Autodesk Inventor part; units mm, degrees
ref_plane "YZ Plane" through (0, 0, 0) normal (1, 0, 0) x (0, 1, 0)
ref_plane "XZ Plane" through (0, 0, 0) normal (0, 1, 0) x (-1, 0, 0)
ref_plane "XY Plane" through (0, 0, 0) normal (0, 0, 1) x (1, 0, 0)
sketch "Sketch1" plane through (0, 0, 0) normal (0, 0, 1) x (1, 0, 0)
  line L0 (-17.5, 17.5) -> (17.5, 17.5)
  line L1 (17.5, 17.5) -> (17.5, -17.5)
  line L2 (17.5, -17.5) -> (-17.5, -17.5)
  line L3 (-17.5, -17.5) -> (-17.5, 17.5)
  line L4 (14.5, 14.5) -> (-14.5, 14.5)
  line L5 (-14.5, 14.5) -> (-14.5, -14.5)
  line L6 (-14.5, -14.5) -> (14.5, -14.5)
  line L7 (14.5, -14.5) -> (14.5, 14.5)
  point P0 (0, 0)
  point P1 (17.5, 0)
  point P2 (0, 17.5)
  dimension "d0" = 35
  dimension "d1" = 35
  dimension "d2" = 3
extrude "Extrusion1" add sketch "Sketch1" against normal mid plane 45
chamfer "Chamfer1" distance 2 angle 45 8 edges at (-17.5, 17.5, 0) (17.5, 17.5, 0) (-14.5, 14.5, 0) (14.5, 14.5, 0) (-14.5, -14.5, 0) (14.5, -14.5, 0) (17.5, -17.5, 0) (-17.5, -17.5, 0)
sketch "Sketch2" plane through (0, 0, 22.5) normal (0, 0, 1) x (1, 0, 0)
  line L0 (15.5, 17.5) -> (-15.5, 17.5)
  line L1 (-12.5, 14.5) -> (12.5, 14.5)
  line L2 (-17.5, 15.5) -> (-15.5, 17.5)
  line L3 (-12.5, 14.5) -> (-14.5, 12.5)
  line L4 (14.5, 12.5) -> (12.5, 14.5)
  line L5 (15.5, 17.5) -> (17.5, 15.5)
  line L6 (-17.5, 15.5) -> (-17.5, -15.5)
  line L7 (-14.5, -12.5) -> (-14.5, 12.5)
  line L8 (-14.5, -12.5) -> (-12.5, -14.5)
  line L9 (-15.5, -17.5) -> (15.5, -17.5)
  line L10 (17.5, -15.5) -> (17.5, 15.5)
  line L11 (-15.5, -17.5) -> (-17.5, -15.5)
  line L12 (12.5, -14.5) -> (-12.5, -14.5)
  point P0 (0, 0)
  point P1 (-15, 15)
  point P2 (15, 15)
  point P3 (15, -15)
  point P4 (-15, -17.5)
  point P5 (-15, -15)
  point P6 (15, -17.5)
  dimension "d8" = 3
  dimension "d9" = 4.2426
  dimension "d10" = 2.1213
  dimension "d11" = 5
  dimension "d12" = 2.5
  dimension "d13" = 2.5
  dimension "d14" = 4.2426
  dimension "d15" = 2.1213
  dimension "d26" = 5
  dimension "d27" = 2.5
  dimension "d28" = 5
  dimension "d29" = 2.5
  dimension "d30" = 2.5
  dimension "d31" = 2.5
  dimension "d64" = 4.2426
hole "Hole1" at (-15, 15, 22.5) at (15, 15, 22.5) at (15, -15, 22.5) at (-15, -15, 22.5) direction (0, 0, -1) diameter 2.459 depth 8.8 tip angle 118
sketch "Sketch4" plane through (0, 0, -22.5) normal (0, 0, -1) x (-1, 0, 0)
  line L0 (15.5, 17.5) -> (-15.5, 17.5)
  line L1 (-12.5, 14.5) -> (12.5, 14.5)
  line L2 (-17.5, 15.5) -> (-15.5, 17.5)
  line L3 (-12.5, 14.5) -> (-14.5, 12.5)
  line L4 (14.5, 12.5) -> (12.5, 14.5)
  line L5 (15.5, 17.5) -> (17.5, 15.5)
  line L6 (-17.5, 15.5) -> (-17.5, -17.5)
  line L7 (-14.5, -12.5) -> (-14.5, 12.5)
  line L8 (-14.5, -12.5) -> (-12.5, -14.5)
  line L9 (-17.5, -17.5) -> (17.5, -17.5)
  line L10 (17.5, -17.5) -> (17.5, 15.5)
  line L11 (-17.5, 15.5) -> (-15.5, 17.5)
  line L12 (-17.5, 15.5) -> (-17.5, -15.5)
  line L13 (-15.5, -17.5) -> (15.5, -17.5)
  line L14 (17.5, -15.5) -> (17.5, 15.5)
  line L15 (15.5, 17.5) -> (17.5, 15.5)
  line L16 (15.5, 17.5) -> (-15.5, 17.5)
  line L17 (-14.5, -12.5) -> (-14.5, 12.5)
  line L18 (-12.5, 14.5) -> (-14.5, 12.5)
  line L19 (-12.5, 14.5) -> (12.5, 14.5)
  line L20 (14.5, 12.5) -> (12.5, 14.5)
  line L21 (14.5, 12.5) -> (14.5, -12.5)
  line L22 (12.5, -14.5) -> (14.5, -12.5)
  line L23 (12.5, -14.5) -> (-12.5, -14.5)
  line L24 (-14.5, -12.5) -> (-12.5, -14.5)
  line L25 (17.5, -15.5) -> (15.5, -17.5)
  line L26 (-15.5, -17.5) -> (-17.5, -15.5)
  point P0 (0, 0)
  point P1 (0, 0)
  point P2 (-15, 15)
  point P3 (15, 15)
  point P4 (15, -15)
  point P5 (-15, -15)
  dimension "d39" = 3
  dimension "d40" = 4.2426
  dimension "d41" = 2.1213
  dimension "d42" = 5
  dimension "d43" = 2.5
  dimension "d44" = 2.5
  dimension "d45" = 4.2426
  dimension "d46" = 2.1213
  dimension "d47" = 5.6569
  dimension "d48" = 5
  dimension "d49" = 2.5
  dimension "d50" = 5
  dimension "d51" = 2.5
  dimension "d52" = 2.5
  dimension "d53" = 2.5
hole "Hole2" at (15, 15, -22.5) at (-15, 15, -22.5) at (-15, -15, -22.5) at (15, -15, -22.5) direction (0, 0, 1) diameter 2.459 depth 8.8 tip angle 118
sketch "Sketch7" plane through (0, 0, 22.5) normal (0, 0, 1) x (1, 0, 0)
  circle A0 centre (0, 0) radius 13.25
  circle A1 centre (15, -15) radius 1.2295
  circle A2 centre (-15, 15) radius 1.2295
  circle A3 centre (15, 15) radius 1.2295
  circle A4 centre (-15, -15) radius 1.2295
  line L0 (15.5, 17.5) -> (17.5, 15.5)
  line L1 (15.5, 17.5) -> (-15.5, 17.5)
  line L2 (-17.5, 15.5) -> (-15.5, 17.5)
  line L3 (-17.5, 15.5) -> (-17.5, -15.5)
  line L4 (-15.5, -17.5) -> (15.5, -17.5)
  line L5 (17.5, -15.5) -> (17.5, 15.5)
  line L6 (14.5, 12.5) -> (14.5, -12.5)
  line L7 (12.5, -14.5) -> (14.5, -12.5)
  line L8 (12.5, -14.5) -> (-12.5, -14.5)
  line L9 (-14.5, -12.5) -> (-12.5, -14.5)
  line L10 (-14.5, -12.5) -> (-14.5, 12.5)
  line L11 (-12.5, 14.5) -> (-14.5, 12.5)
  line L12 (-12.5, 14.5) -> (12.5, 14.5)
  line L13 (14.5, 12.5) -> (12.5, 14.5)
  line L14 (-15.5, -17.5) -> (-17.5, -15.5)
  line L15 (17.5, -15.5) -> (15.5, -17.5)
  dimension "d61" = 26.5
extrude "Extrusion2" add sketch "Sketch7" against normal blind 35 contours L6 L7 L8 L9 L10 L11 L12 L13
properties part number "Cover for servo motor 250 W" material "Stainless Steel"
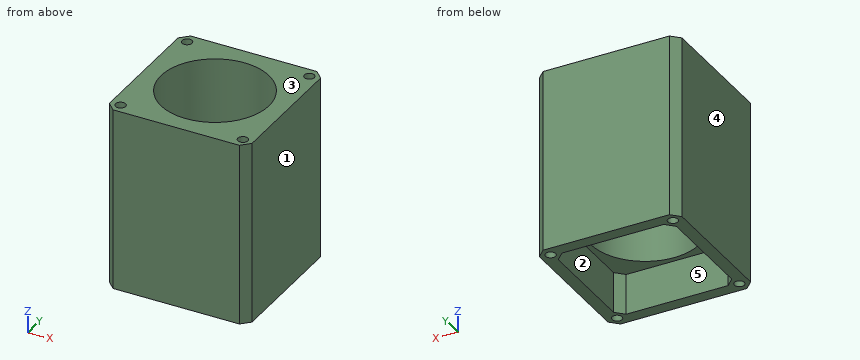
Design review of the part built by this model. Coordinates are the model's own, in mm. Face numbers are marked on the shaded views. A direction names the side the tool comes from. Coordinates: 2 decimals unless noted, no trailing zeros. Order: outer loops, then holes, each group sorted by start corner. A loop starts at its lowest first (then second) coordinate and runs counter-clockwise, first axis right, second up. Notation, with made-up numbers: (31, 66.5) - (84, 66.5) arc R24 cw to (84, 89.5) - close; hole circle Ø2 at (-20.75, 61). An arc over 180 degrees is marked (long way). Answer in a Markdown table with one row per item.
(1) Consider section A-A on y = 0. State the section outline as (x, z) points, plus the area to 4 significant figures.
Checked values:
| item | result |
|---|---|
| outline | (-17.5, -22.5) - (-14.5, -22.5) - (-14.5, -12.5) - (-13.25, -12.5) - (-13.25, 22.5) - (-17.5, 22.5) - close; (13.25, -12.5) - (14.5, -12.5) - (14.5, -22.5) - (17.5, -22.5) - (17.5, 22.5) - (13.25, 22.5) - close |
| area | 357.5 mm^2 |
(2) Wall thickness on line 1 along X through (y, z) = (-15, 17.5); line 2 along Y through (x, z) = (11.5, -18): over which ranges is each line inside the solid? List them lowest first. Write a range as from..to.
Checked values:
| item | result |
|---|---|
| line 1 | -17.5..-16.23, -13.77..13.77, 16.23..17.5 |
| line 2 | -17.5..-14.5, 14.5..17.5 |
(3) Consider section C-C on z = 6.5. State the section outline as (x, y) points.
Checked values:
| item | result |
|---|---|
| outline | (-17.5, -15.5) - (-15.5, -17.5) - (15.5, -17.5) - (17.5, -15.5) - (17.5, 15.5) - (15.5, 17.5) - (-15.5, 17.5) - (-17.5, 15.5) - close; hole circle Ø26.5 at (0, 0) |
(4) The part is to be moulded in two halves that separate along X. For the marked faces 3, 4 and 5, say which applies: released by +X, released by -X, zero draft, split by the parting line, or undercut.
Checked values:
| item | result |
|---|---|
| face 3 | zero draft |
| face 4 | released by -X |
| face 5 | undercut |
(5) For the marked faces 1 and 2, list the 3-axis set-ups (+Z, -Z, +X, -X, +Y, -Y) from which the entire face can be reached by the end or side of a thin tool; tool diameter is ignored.
Checked values:
| item | result |
|---|---|
| face 1 | +Z, -Z, +X, +Y, -Y |
| face 2 | -Z |
(6) Clearance check with flat-ended pins moving along their axes: pin 1 (6 mm diameter, centred on x = 2, y = 12.5, fed in from -Z); pin 2 (14.5 mm diameter, centred on x = 7, y = 2.5, fed in from -Z); pin 3 (1.5 mm diameter, centred on x = -15, y = -15, fed in from -Z); pin 4 (1.5 mm diameter, centred on x = 15, y = -15, fed in from +Z). State where each tip first meets the part, or that it passes through.
Checked values:
| item | result |
|---|---|
| pin 1 | z = -22.5 |
| pin 2 | z = -12.5 |
| pin 3 | z = -13.41 |
| pin 4 | z = 13.41 |
